Read the model definition and answer for the solid it produces. Units are mm, in the model's axes. Round coordinates to 2 decimals unless told otherwise and drop trailing zeros. Order: outer loops, then holes, each group sorted by start corner. A loop starts at its lowest first (then second) coordinate and runs counter-clockwise, first axis right, second up. Notation, with made-up numbers: (57.5, -5.5) - (80.5, -5.5) arc R19 ccw to (80.5, 15.5) - close; hole circle Ø11 at (26.5, 19). An arc over 180 degrees is marked (long way). One line per question, with ' | ' between items. Start each with the question number.
1) The part is cut by section C-C, the plane x = 29. Give the vertices of the cut face in (y, z), plus the area to 3 significant figures.
2) Straight lines are drawn through the part: line 1 (Y direction, x = 3, z = 7.4); line 2 (X direction, y = -4.25, z = 7.25); line 3 (X direction, y = -3.5, z = 8.35). For each, find the intervals that lie inside material, in ascending order. Write a range as from..to.
3) The part is cut by section A-A, the plane x = 131. Give the vertices of the cut face in (y, z), plus the area to 3 significant figures.
4) The part is cut by section B-B, the plane z = 8.15. Count the separate pieces of the cut face and the enclosed holes in it, plus the area to 3 significant figures.
from build123d import *

# Parameters (mm, degrees)
SKETCH2_W               = 160
SKETCH2_H               = 20
BOSS_EXTRUDE1_DEPTH     = 3.2
CUT_EXTRUDE1_DEPTH      = 162.276904732
CUT_EXTRUDE1_DEPTH_BACK = 162.276904732
SKETCH5_R               = 4
SKETCH5_R_2             = 2
SKETCH6_R               = 1.5
CUT_EXTRUDE2_DEPTH      = 10
CUT_EXTRUDE3_DEPTH      = 162.276904732
CUT_EXTRUDE3_DEPTH_BACK = 162.276904732
SKETCH7_R               = 1
SKETCH8_R               = 1.5
CUT_EXTRUDE4_DEPTH      = 10
SKETCH9_R               = 1.5
CUT_EXTRUDE5_DEPTH      = 10


with BuildPart() as part:
    # Sketch2 → Boss-Extrude1 (new body)
    with BuildSketch(Plane(origin=(0, -10, 10), x_dir=(1, 0, 0), z_dir=(0, 0, -1))):
        with Locations((80, 0)):
            Rectangle(SKETCH2_W, SKETCH2_H)
    extrude(amount=BOSS_EXTRUDE1_DEPTH)

    # Sketch5 → Cut-Extrude1 (cut, two sides: drawn at the far end of the back side and taken through both)
    with BuildSketch(Plane.XY.offset(10).offset(-CUT_EXTRUDE1_DEPTH_BACK)):
        with Locations((131, -7)):
            Circle(SKETCH5_R)
        with Locations((29, -7)):
            Circle(SKETCH5_R_2)
    extrude(amount=CUT_EXTRUDE1_DEPTH + CUT_EXTRUDE1_DEPTH_BACK, mode=Mode.SUBTRACT)

    # Sketch6 → Cut-Extrude2 (cut)
    with BuildSketch(Plane.XY.offset(10)):
        with Locations((96, -11)):
            Circle(SKETCH6_R)
        with Locations((64, -11)):
            Circle(SKETCH6_R)
    extrude(amount=-CUT_EXTRUDE2_DEPTH, mode=Mode.SUBTRACT)

    # Sketch7 → Cut-Extrude3 (cut, two sides: drawn at the far end of the back side and taken through both)
    with BuildSketch(Plane.XY.offset(10).offset(-CUT_EXTRUDE3_DEPTH_BACK)):
        with Locations((3, -15)):
            Circle(SKETCH7_R)
        with Locations((3, -5)):
            Circle(SKETCH7_R)
    extrude(amount=CUT_EXTRUDE3_DEPTH + CUT_EXTRUDE3_DEPTH_BACK, mode=Mode.SUBTRACT)

    # Sketch8 → Cut-Extrude4 (cut)
    with BuildSketch(Plane.XY.offset(10)):
        with Locations((146, -3)):
            Circle(SKETCH8_R)
        with Locations((116, -3)):
            Circle(SKETCH8_R)
    extrude(amount=-CUT_EXTRUDE4_DEPTH, mode=Mode.SUBTRACT)

    # Sketch9 → Cut-Extrude5 (cut)
    with BuildSketch(Plane(origin=(0, 0, 6.8), x_dir=(-1, 0, 0), z_dir=(0, 0, -1))):
        with Locations((-20, -7)):
            Circle(SKETCH9_R)
        with Locations((-38, -7)):
            Circle(SKETCH9_R)
    extrude(amount=-CUT_EXTRUDE5_DEPTH, mode=Mode.SUBTRACT)


solid = part.part
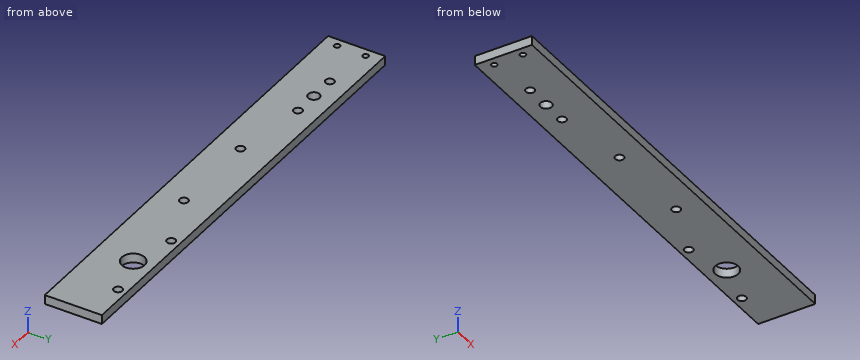
Values:
1) outline: (-20, 6.8) - (-9, 6.8) - (-9, 10) - (-20, 10) - close; (-5, 6.8) - (0, 6.8) - (0, 10) - (-5, 10) - close | area: 51.2 mm^2
2) line 1: y = -20..-16, -14..-6, -4..0 | line 2: x = 0..2.34, 3.66..115.17, 116.83..128.1, 133.9..145.17, 146.83..160 | line 3: x = 0..114.59, 117.41..129.06, 132.94..144.59, 147.41..160
3) outline: (-20, 6.8) - (-11, 6.8) - (-11, 10) - (-20, 10) - close; (-3, 6.8) - (0, 6.8) - (0, 10) - (-3, 10) - close | area: 38.4 mm^2
4) separate pieces: 1 | enclosed holes: 10 | area: 3,090 mm^2
